The model under review builds one solid part; all positions refer to its coordinate system, in mm. Face numbers are marked on the shaded views. Coordinates: 2 decimals unless noted, no trailing zeros. Loops run counter-clockwise (first coordinate to the right, second up) from the corner with the lowest first, then second, coordinate; pieces in that order, holes last. Notation, with made-up numbers: M 73.25,45 L 112.25,45 A9 cw 112.25,55 Z; hole C 46,87.25 d9. An arc over 180 degrees is marked long. Return JSON: item names as keys, results as strings.
Autodesk Inventor part; units mm, degrees
ref_plane "YZ Plane" through (0, 0, 0) normal (1, 0, 0) x (0, 1, 0)
ref_plane "XZ Plane" through (0, 0, 0) normal (0, 1, 0) x (-1, 0, 0)
ref_plane "XY Plane" through (0, 0, 0) normal (0, 0, 1) x (1, 0, 0)
sketch "スケッチ1" plane through (0, 0, 0) normal (1, 0, 0) x (0, 1, 0)
  circle A0 centre (0, 0) radius 17.5
  dimension "d0" = 35
extrude "押し出し1" add sketch "スケッチ1" along normal blind 6
sketch "スケッチ2" plane through (6, 0, 0) normal (1, 0, 0) x (0, 0, -1)
  circle A0 centre (0, 0) radius 13.5
  point P0 (13.5, 0)
  point P1 (6.75, 11.6913)
  point P2 (-6.75, 11.6913)
  point P3 (-13.5, 0)
  point P4 (-6.75, -11.6913)
  point P5 (6.75, -11.6913)
  dimension "d3" = 27
  dimension "d6" = 360
hole "穴1" at (6, 0, -13.5) at (6, 11.6913, -6.75) at (6, 11.6913, 6.75) at (6, 0, 13.5) at (6, -11.6913, 6.75) at (6, -11.6913, -6.75) direction (-1, 0, 0) diameter 3.2 end through all
properties part number "link5_plate1" material "ABS プラスチック"
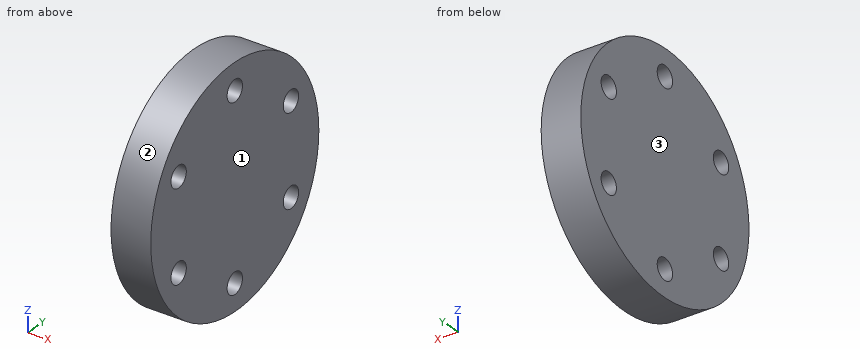
1. Add section C-C on z = -13.5. Give the boundary of the cut face in (x, y).
Check values:
{"outline": "M 0,-11.14 L 6,-11.14 L 6,-1.6 L 0,-1.6 Z; M 0,1.6 L 6,1.6 L 6,11.14 L 0,11.14 Z"}
2. To check wall thickness, follow line 1 (Z direction, x = 3.95, y = 0); line 2 (Y direction, x = 3.8, z = 6.75); line 3 (Z direction, x = 1.1, y = -12). State the ranges of each line that lie inside material, in increasing order.
Check values:
{"line 1": "-17.5 to -15.1, -11.9 to 11.9, 15.1 to 17.5", "line 2": "-16.15 to -13.29, -10.09 to 10.09, 13.29 to 16.15", "line 3": "-12.74 to -8.32, -5.18 to 5.18, 8.32 to 12.74"}
3. Insertion check: pin 1 Ø3.5 at (y, z) = (11.69, -6.75) entering from +X; pin 2 Ø1.5 at (x, z) = (1.5, -10.5) entering from -Y; pin 3 Ø1 at (x, y) = (3, -11) entering from +Z. Each pin has a flat end and moves straight along its axis. Give the tip position at first contact, or say it passes through.
Check values:
{"pin 1": "x = 6", "pin 2": "y = -14.53", "pin 3": "z = 14"}
4. Add section A-A on y = 0. Give the boundary of the cut face in (x, z).
Check values:
{"outline": "M 0,-17.5 L 6,-17.5 L 6,-15.1 L 0,-15.1 Z; M 0,-11.9 L 6,-11.9 L 6,11.9 L 0,11.9 Z; M 0,15.1 L 6,15.1 L 6,17.5 L 0,17.5 Z"}
5. Add section B-B on z = -7.5. Give the boundary of the cut face in (x, y), plus the area to 3 significant figures.
Check values:
{"outline": "M 0,-15.81 L 6,-15.81 L 6,-13.1 L 0,-13.1 Z; M 0,-10.28 L 6,-10.28 L 6,10.28 L 0,10.28 Z; M 0,13.1 L 6,13.1 L 6,15.81 L 0,15.81 Z", "area": "156 mm²"}
6. The part is to be moulded in two halves that separate along X. For the marked faces 1, 2 and 3, say which applies: released by +X, released by -X, zero draft, split by the parting line, or undercut.
Check values:
{"face 1": "released by +X", "face 2": "zero draft", "face 3": "released by -X"}
7. Add section D-D on x = 5.4. Give the boundary of the cut face in (y, z).
Check values:
{"outline": "C 0,0 d35; hole C -11.69,-6.75 d3.2; hole C -11.69,6.75 d3.2; hole C 0,-13.5 d3.2; hole C 0,13.5 d3.2; hole C 11.69,-6.75 d3.2; hole C 11.69,6.75 d3.2"}
